Check sheet for the modelled part. Datum: model origin and axes. Units: mm. A direction names the side the tool comes from. Round coordinates to 2 decimals unless told otherwise and drop trailing zeros. Loops run counter-clockwise (first coordinate to the right, second up) from the corner with the lowest first, then second, coordinate; pieces in that order, holes last. Notation, with made-up numbers: M 44,-1 L 86,-1 A10 ccw 86,7 Z; hole C -25.75,64.25 d4. An arc over 180 degrees is marked long. Write item = value, one per line. Start each with the question number.
(1) Mould release check, pull along X, two halves, no side actions. Record for faces 4 (the face through (-2, 2, 8.2)), 5 (the face through (4.83, 1.52, 4.07)), 6 (the face through (0, 0, 6.5)): pulls with the +X half, pulls with the -X half, needs draft (parallel to the pull), parting line crosses it, or undercut.
(2) Cross-section at C-C on z = 9. Record the boundary of the cut face in (x, y), plus the area to 3 significant figures.
(3) Cross-section at A-A on x = 0. Record the boundary of the cut face in (y, z) (3 decimals), plus the area to 3 significant figures.
(4) Set-up check for faces 1 (the face through (-0.5, -2.4, 9.1)), 2 (the face through (2.28, -0.72, 2.63)), 3 (the face through (0, -2, 10.09)): record each of +Z, -Z, +X, -X, +Y, -Y from which the full face is reachable in a straight line by a thin tool's end or side.
(5) Scan lines: L1, parallel to Y at x = 0, z = 8.9; L2, parallel to Y at x = 0, z = 4.25 (3 decimals); L3, parallel to X at y = -1.5, z = 2.5. Record each from-to range of solid material in increasing order. Write a range as from..to.
(6) Cross-section at D-D on z = 7.75. Record the boundary of the cut face in (x, y), plus the area to 3 significant figures.
(7) Go/stop test with flat-tipped pins: P1, Ø4, axis at y = -2.5, z = 5, coming from the -X side; P2, Ø1.5, axis at y = 3.5, z = 2, coming from the -X side; P3, Ø1.5, axis at x = -3, y = -3, coming from the -Z side. Record where each tip stops, or that it passes through.
from build123d import *

# Parameters (mm, degrees)
F0_R     = 5.065
F1_DEPTH = 8.2
F2_R     = 1.835
F3_R     = 2.45
F4_DEPTH = 1.89
F5_R     = 1.58
F6_DEPTH = 1.89
F7_R     = 3.23
F7_R_2   = 2.39
F8_DEPTH = 1.35
F9_DEPTH = 6.5


with BuildPart() as f1:
    # F0 (on Top) → F1 (new body)
    with BuildSketch(Plane.XY):
        Circle(F0_R)
    extrude(amount=F1_DEPTH)

    # F2
    f2_edges = [f1.edges().sort_by_distance(p)[0] for p in [
        (-5.065, 0, 8.2),
        (-5.065, 0, 0),
    ]]
    fillet(f2_edges, radius=F2_R)

    # F3 (on face) → F4 (join)
    with BuildSketch(Plane.XY.offset(8.2)):
        Circle(F3_R)
    extrude(amount=F4_DEPTH)

    # F5 (on face) → F6 (cut)
    with BuildSketch(Plane.XY.offset(10.09)):
        Circle(F5_R)
    extrude(amount=-F6_DEPTH, mode=Mode.SUBTRACT)

    # F7 (on face) → F8 (join)
    with BuildSketch(Plane(origin=(0, 0, 0), x_dir=(1, 0, 0), z_dir=(0, 0, -1))):
        Circle(F7_R)
        Circle(F7_R_2, mode=Mode.SUBTRACT)
    extrude(amount=F8_DEPTH)

    # F9 (cut): a face of the model
    f9_faces = [f1.faces().sort_by_distance(p)[0] for p in [
        (0, 0, 0),
    ]]
    extrude(f9_faces, amount=-F9_DEPTH, mode=Mode.SUBTRACT)


solid = f1.part
Result:
q1.face_4 = needs draft
q1.face_5 = parting line crosses it
q1.face_6 = undercut
q2.outline = C 0,0 d4.9; hole C 0,0 d3.16
q2.area = 11.0 mm^2
q3.outline = M -5.065,1.835 A1.835 ccw -3.23,0 L -3.23,-1.35 L -2.39,-1.35 L -2.39,6.5 L 2.39,6.5 L 2.39,-1.35 L 3.23,-1.35 L 3.23,0 A1.835 ccw 5.065,1.835 L 5.065,6.365 A1.835 ccw 3.23,8.2 L 2.45,8.2 L 2.45,10.09 L 1.58,10.09 L 1.58,8.2 L -1.58,8.2 L -1.58,10.09 L -2.45,10.09 L -2.45,8.2 L -3.23,8.2 A1.835 ccw -5.065,6.365 Z
q3.area = 54.7 mm^2
q4.face_1 = +Z
q4.face_2 = -Z
q4.face_3 = +Z, +X, -X, +Y, -Y
q5.L1 = -2.45..-1.58, 1.58..2.45
q5.L2 = -5.065..-2.39, 2.39..5.065
q5.L3 = -4.84..-1.86, 1.86..4.84
q6.outline = C 0,0 d8.87
q6.area = 61.8 mm^2
q7.P1 = -5.04
q7.P2 = -4.25
q7.P3 = 0.02
